Print and shaded views of the part. All mm, measured from the part's lowest x, y and z. A direction names the side the tool comes from. Round coordinates to 2 decimals unless told otherwise and drop trailing zeros. Loops run counter-clockwise (first coordinate to the right, second up) from the corner with the lowest first, then second, coordinate; pieces in that order, holes last. Notation, with made-up numbers: (-9, 54.5) - (48, 54.5) arc R23 cw to (48, 88.5) - close; hole circle Ø7 at (-25, -29.5). An arc over 180 degrees is marked (long way). Use one line per item in the form item = value.
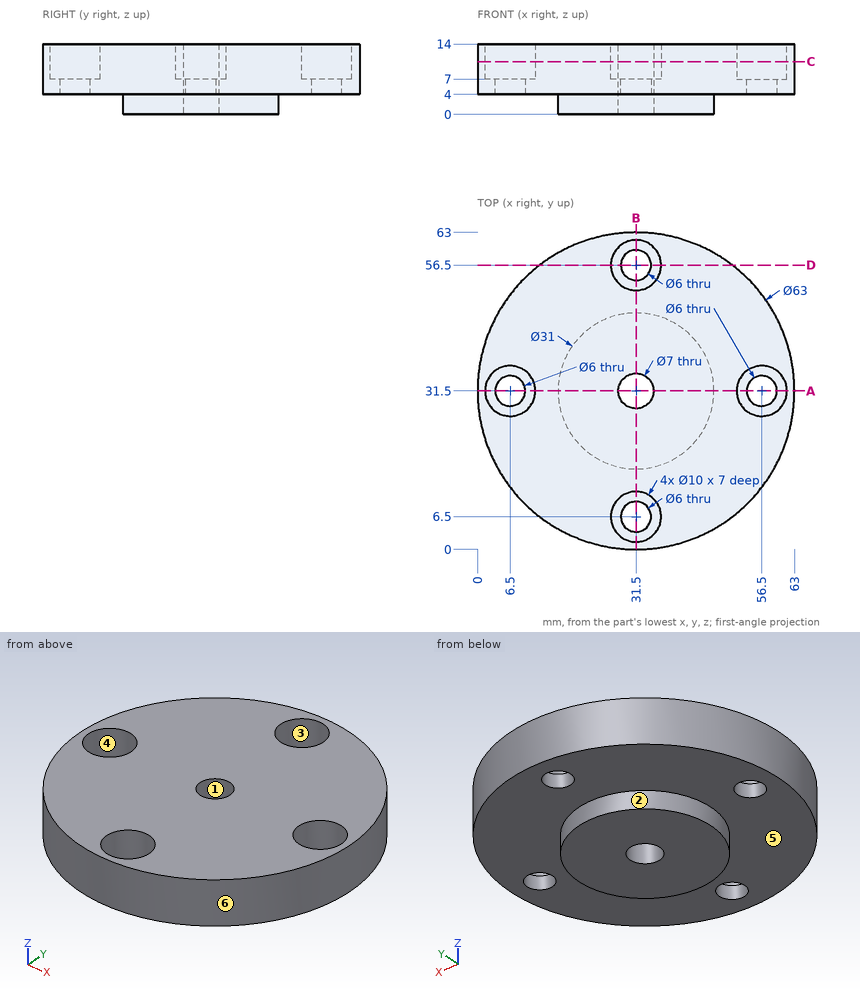
1) Slice it at D-D (y = 56.5). Write the cut outline in (x, z).
Report:
outline = (12.34, 4) - (28.5, 4) - (28.5, 7) - (26.5, 7) - (26.5, 14) - (12.34, 14) - close; (34.5, 4) - (50.66, 4) - (50.66, 14) - (36.5, 14) - (36.5, 7) - (34.5, 7) - close
2) Flat gauge pins, fed straight in: pin 1 (9.5 mm diameter, centred on x = 31.5, y = 56.5, fed in from -Z); pin 2 (1 mm diameter, centred on x = 23, z = 3, fed in from -Y); pin 3 (3.5 mm diameter, centred on x = 31.5, y = 6.5, fed in from +Z); pin 4 (1 mm diameter, centred on y = 46, z = 4.5, fed in from +X). Where does each tip first touch, or does it go through?
Report:
pin_1 = 4
pin_2 = 18.22
pin_3 = through
pin_4 = 59.72
3) Tool access for the marked faces 1, 2 and 3: list every direction of +Z, -Z, +X, -X, +Y, -Y with a clear straight run to the whole face (end or side of a thin tool).
Report:
face_1 = +Z, -Z
face_2 = -Z
face_3 = +Z
4) Slice it at A-A (y = 31.5). Write the cut outline in (x, z).
Report:
outline = (0, 4) - (3.5, 4) - (3.5, 7) - (1.5, 7) - (1.5, 14) - (0, 14) - close; (9.5, 4) - (16, 4) - (16, 0) - (28, 0) - (28, 14) - (11.5, 14) - (11.5, 7) - (9.5, 7) - close; (35, 0) - (47, 0) - (47, 4) - (53.5, 4) - (53.5, 7) - (51.5, 7) - (51.5, 14) - (35, 14) - close; (59.5, 4) - (63, 4) - (63, 14) - (61.5, 14) - (61.5, 7) - (59.5, 7) - close
5) Slice it at C-C (z = 10.5). Write the cut outline in (x, y).
Report:
outline = circle Ø63 at (31.5, 31.5); hole circle Ø10 at (6.5, 31.5); hole circle Ø10 at (31.5, 6.5); hole circle Ø10 at (31.5, 56.5); hole circle Ø7 at (31.5, 31.5); hole circle Ø10 at (56.5, 31.5)
6) Two-plate mould, pull along Y, no slides. Class the marked faces 4, 5 and 6: +Y half, -Y half, draft (parallel to the pull), parting line (faces both ways), or undercut.
Report:
face_4 = undercut
face_5 = draft
face_6 = parting line
7) Drill centre lines: probe 1 along Y at (x, z) = (31.5, 9.5); probe 2 along Y at (x, z) = (32, 6.25); probe 3 along Z at (x, y) = (14, 54.5). Where is each one in solid material? Low to high.
Report:
probe_1 = 0 to 1.5, 11.5 to 28, 35 to 51.5, 61.5 to 63
probe_2 = 0 to 3.54, 9.46 to 28.04, 34.96 to 53.54, 59.46 to 63
probe_3 = 4 to 14
